Input: part model. Units: mm. Frame: model coordinates. A direction names the side the tool comes from. Coordinates: 2 decimals unless noted, no trailing zeros. Order: outer loops, then holes, each group sorted by start corner. A loop starts at its lowest first (then second) coordinate and runs counter-clockwise, first axis right, second up. Notation, with made-up numbers: (48, 63.25) -> (66, 63.25) arc R28 ccw to (66, 95.25) -> close; hole circle Ø11 at (-1, 35.5). An arc over 180 degrees is marked (long way). Write each question's results on one line, items separated by ' | '.
Autodesk Inventor part; units mm, degrees
ref_plane "YZ Plane" through (0, 0, 0) normal (1, 0, 0) x (0, 1, 0)
ref_plane "XZ Plane" through (0, 0, 0) normal (0, 1, 0) x (-1, 0, 0)
ref_plane "XY Plane" through (0, 0, 0) normal (0, 0, 1) x (1, 0, 0)
sketch "Sketch1" plane through (0, 0, 0) normal (0, 0, 1) x (1, 0, 0)
  line L0 (-20, 20) -> (20, 20)
  line L1 (20, 20) -> (20, -20)
  line L2 (20, -20) -> (-20, -20)
  line L3 (-20, -20) -> (-20, 20)
  line L4 (-20, 20) -> (20, -20) construction
  line L5 (20, 20) -> (-20, -20) construction
  line L6 (20, -5) -> (30, -5)
  line L7 (30, -5) -> (30, 5)
  line L8 (30, 5) -> (20, 5)
  line L9 (20, 5) -> (20, -5)
  line L10 (-20, -5) -> (-30, -5)
  line L11 (-30, -5) -> (-30, 5)
  line L12 (-30, 5) -> (-20, 5)
  line L13 (-20, 5) -> (-20, -5)
  circle A0 centre (-25, 0) radius 2.75
  circle A1 centre (25, 0) radius 2.75
  point P0 (0, 0)
  point P1 (30, 0)
  point P2 (20, 0)
  point P3 (-25, 5)
  point P4 (25, 5)
  dimension "d0" = 40
  dimension "d1" = 40
  dimension "d2" = 10
  dimension "d3" = 10
  dimension "d4" = 10
  dimension "d5" = 5.5
  dimension "d6" = 5.5
extrude "Extrusion1" add sketch "Sketch1" along normal blind 10
properties part number "cap5V"
(1) Pin query (flat end, axial travel): P1, Ø3, axis at y = 9.5, z = 5, coming from the +X side; P2, Ø8, axis at x = 11, y = 4.5, coming from the -Z side; P3, Ø3, axis at y = -11, z = 6, coming from the -X side; P4, Ø1.5, axis at x = -22, z = 7, coming from the +Y side. Return the tip coordinate at first contact, or that it passes through.
Return value:
P1: x = 20 | P2: z = 0 | P3: x = -20 | P4: y = 5
(2) Cut plane B-B, the plane y = 0. Return loops of the section in (x, z).
Return value:
outline: (-30, 0) -> (-27.75, 0) -> (-27.75, 10) -> (-30, 10) -> close; (-22.25, 0) -> (22.25, 0) -> (22.25, 10) -> (-22.25, 10) -> close; (27.75, 0) -> (30, 0) -> (30, 10) -> (27.75, 10) -> close
(3) Cut plane C-C, the plane z = 6.75. Return loops of the section in (x, y), plus the area to 3 significant figures.
Return value:
outline: (-30, -5) -> (-20, -5) -> (-20, -20) -> (20, -20) -> (20, -5) -> (30, -5) -> (30, 5) -> (20, 5) -> (20, 20) -> (-20, 20) -> (-20, 5) -> (-30, 5) -> close; hole circle Ø5.5 at (-25, 0); hole circle Ø5.5 at (25, 0) | area: 1,750 mm2
(4) Cut plane D-D, the plane y = 8. Return loops of the section in (x, z).
Return value:
outline: (-20, 0) -> (20, 0) -> (20, 10) -> (-20, 10) -> close
(5) Line query: line 1 along X through (y, z) = (1.5, 3); line 2 along Y through (x, z) = (25, 7.5); line 3 along X through (y, z) = (-0.5, 4.75). Output: solid intervals per line, ascending. Write a range as from..to.
Return value:
line 1: -30..-27.3, -22.7..22.7, 27.3..30 | line 2: -5..-2.75, 2.75..5 | line 3: -30..-27.7, -22.3..22.3, 27.7..30
(6) Mould query, pull axis Y, two halves, no side actions, for faces 6 (the face through (-25, 5, 5)), 7 (the face through (-27.747, -0.121, 4.93)), 8 (the face through (20, 13, 5)), 9 (the face through (0, -20, 5)). Classes: +Y half, -Y half, draft (parallel to the pull), parting line (faces both ways), or undercut.
Return value:
face 6: +Y half | face 7: undercut | face 8: draft | face 9: -Y half
(7) Reachability of faces 1 (the face through (25, -5, 5)), 2 (the face through (25, 5, 5)), 3 (the face through (-20, 12, 5)), 4 (the face through (-20, -13, 5)), 5 (the face through (0, 20, 5)) from +Z, -Z, +X, -X, +Y, -Y: full face, straight path, thin tool, end or side. Return the list, or none.
Return value:
face 1: +Z, -Z, +X, -Y | face 2: +Z, -Z, +X, +Y | face 3: +Z, -Z, -X, +Y | face 4: +Z, -Z, -X, -Y | face 5: +Z, -Z, +X, -X, +Y
(8) Cut plane A-A, the plane x = -25. Return loops of the section in (y, z), plus the area to 3 significant figures.
Return value:
outline: (-5, 0) -> (-2.75, 0) -> (-2.75, 10) -> (-5, 10) -> close; (2.75, 0) -> (5, 0) -> (5, 10) -> (2.75, 10) -> close | area: 45.0 mm2
